For this review, take the finished solid that the model builds, in its own axes (mm). Give positions to 0.01 mm unless a question says otherwise; leave off trailing zeros. Write each loop counter-clockwise with the first axis right and the second up, starting at its lowest first coordinate (ties: lowest second). Pieces come first, ordered by that corner, then holes. Notation, with made-up numbers: (-33.5, 32.5) -> (14.5, 32.5) arc R29 ccw to (14.5, 65.5) -> close; hole circle Ø1 at (43, -15.5). An arc over 180 degrees is marked (long way). Answer as CSV lines item,"result".
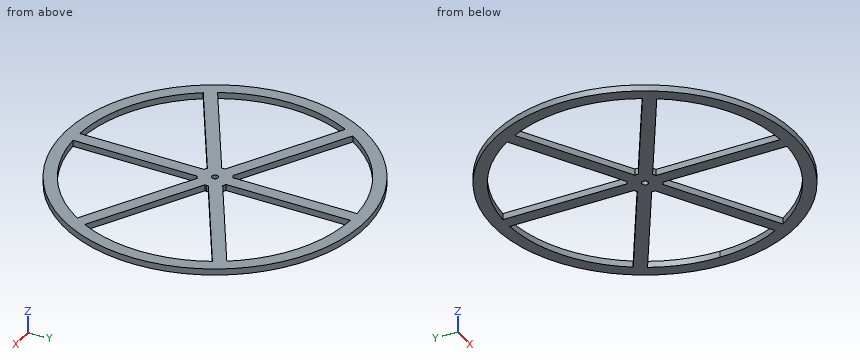
```python
from build123d import *

# Parameters (mm, degrees)
F0_R     = 76.2
F0_R_2   = 1.5875
F1_DEPTH = 3.175


with BuildPart() as f1:
    # F0 (on Top) → F1 (new body)
    with BuildSketch(Plane.XY):
        Circle(F0_R)
        with BuildLine():
            ThreePointArc((62.016851, 32.139271), (67.863464, 16.540035), (69.85, 0))
            ThreePointArc((69.85, 0), (67.863464, -16.540035), (62.016851, -32.139271))
            ThreePointArc((62.016851, -32.139271), (60.491874, -34.925), (58.841851, -37.638532))
            ThreePointArc((58.841851, -37.638532), (34.925, -60.491874), (3.175, -69.777804))
            ThreePointArc((3.175, -69.777804), (0, -69.85), (-3.175, -69.777804))
            ThreePointArc((-3.175, -69.777804), (-34.925, -60.491874), (-58.841851, -37.638532))
            ThreePointArc((-58.841851, -37.638532), (-60.491874, -34.925), (-62.016851, -32.139271))
            ThreePointArc((-62.016851, -32.139271), (-69.85, 0), (-62.016851, 32.139271))
            ThreePointArc((-62.016851, 32.139271), (-60.491874, 34.925), (-58.841851, 37.638532))
            ThreePointArc((-58.841851, 37.638532), (-34.925, 60.491874), (-3.175, 69.777804))
            ThreePointArc((-3.175, 69.777804), (0, 69.85), (3.175, 69.777804))
            ThreePointArc((3.175, 69.777804), (34.925, 60.491874), (58.841851, 37.638532))
            ThreePointArc((58.841851, 37.638532), (60.491874, 34.925), (62.016851, 32.139271))
        make_face(mode=Mode.SUBTRACT)
        with BuildLine():
            Line((-4.712695, 6.38705), (-58.841851, 37.638532))
            ThreePointArc((-58.841851, 37.638532), (-60.491874, 34.925), (-62.016851, 32.139271))
            Line((-62.016851, 32.139271), (-7.887695, 0.887789))
            ThreePointArc((-7.887695, 0.887789), (-6.874077, 3.96875), (-4.712695, 6.38705))
        make_face()
        with BuildLine():
            ThreePointArc((-62.016851, -32.139271), (-60.491874, -34.925), (-58.841851, -37.638532))
            Line((-58.841851, -37.638532), (-4.712695, -6.38705))
            ThreePointArc((-4.712695, -6.38705), (-6.874077, -3.96875), (-7.887695, -0.887789))
            Line((-7.887695, -0.887789), (-62.016851, -32.139271))
        make_face()
        with BuildLine():
            ThreePointArc((7.9375, 0), (7.925039, 0.444592), (7.887695, 0.887789))
            ThreePointArc((7.887695, 0.887789), (6.874077, 3.96875), (4.712695, 6.38705))
            ThreePointArc((4.712695, 6.38705), (3.96875, 6.874077), (3.175, 7.274839))
            Line((3.175, 7.274839), (-3.175, 7.274839))
            ThreePointArc((-3.175, 7.274839), (-3.96875, 6.874077), (-4.712695, 6.38705))
            ThreePointArc((-4.712695, 6.38705), (-6.874077, 3.96875), (-7.887695, 0.887789))
            ThreePointArc((-7.887695, 0.887789), (-7.9375, 0), (-7.887695, -0.887789))
            ThreePointArc((-7.887695, -0.887789), (-6.874077, -3.96875), (-4.712695, -6.38705))
            ThreePointArc((-4.712695, -6.38705), (-3.96875, -6.874077), (-3.175, -7.274839))
            ThreePointArc((-3.175, -7.274839), (0, -7.9375), (3.175, -7.274839))
            ThreePointArc((3.175, -7.274839), (3.96875, -6.874077), (4.712695, -6.38705))
            ThreePointArc((4.712695, -6.38705), (6.874077, -3.96875), (7.887695, -0.887789))
            ThreePointArc((7.887695, -0.887789), (7.925039, -0.444592), (7.9375, 0))
        make_face()
        Circle(F0_R_2, mode=Mode.SUBTRACT)
        with BuildLine():
            ThreePointArc((-3.175, -69.777804), (0, -69.85), (3.175, -69.777804))
            Line((3.175, -69.777804), (3.175, -7.274839))
            ThreePointArc((3.175, -7.274839), (0, -7.9375), (-3.175, -7.274839))
            Line((-3.175, -7.274839), (-3.175, -69.777804))
        make_face()
        with BuildLine():
            ThreePointArc((58.841851, -37.638532), (60.491874, -34.925), (62.016851, -32.139271))
            Line((62.016851, -32.139271), (7.887695, -0.887789))
            ThreePointArc((7.887695, -0.887789), (6.874077, -3.96875), (4.712695, -6.38705))
            Line((4.712695, -6.38705), (58.841851, -37.638532))
        make_face()
        with BuildLine():
            Line((7.887695, 0.887789), (62.016851, 32.139271))
            ThreePointArc((62.016851, 32.139271), (60.491874, 34.925), (58.841851, 37.638532))
            Line((58.841851, 37.638532), (4.712695, 6.38705))
            ThreePointArc((4.712695, 6.38705), (6.874077, 3.96875), (7.887695, 0.887789))
        make_face()
        with BuildLine():
            Line((3.175, 7.274839), (3.175, 69.777804))
            ThreePointArc((3.175, 69.777804), (0, 69.85), (-3.175, 69.777804))
            Line((-3.175, 69.777804), (-3.175, 7.274839))
            ThreePointArc((-3.175, 7.274839), (0, 7.9375), (3.175, 7.274839))
        make_face()
        with BuildLine():
            Line((-3.175, 7.274839), (3.175, 7.274839))
            ThreePointArc((3.175, 7.274839), (0, 7.9375), (-3.175, 7.274839))
        make_face()
    extrude(amount=F1_DEPTH)


solid = f1.part
```
Q1. Add section C-C (z = 2.5). State how many separate pieces and enclosed holes the cut face has, plus the area to 3 significant figures.
Answer block:
separate pieces,"1"
enclosed holes,"7"
area,"5,470 mm2"
Q2. Add section D-D (y = -52.5). Write out the cut boundary in (x, z) (3 decimals), plus the area to 3 significant figures.
Answer block:
outline,"(-55.229, 0) -> (-46.074, 0) -> (-46.074, 3.175) -> (-55.229, 3.175) -> close; (-3.175, 0) -> (3.175, 0) -> (3.175, 3.175) -> (-3.175, 3.175) -> close; (46.074, 0) -> (55.229, 0) -> (55.229, 3.175) -> (46.074, 3.175) -> close"
area,"78.3 mm2"
Q3. Clearance check with flat-ended pins moving along their axes: pin 1 (1.5 mm diameter, centred on y = 48.5, z = 2.5, fed in from +X); pin 2 (1.6 mm diameter, centred on y = -41.5, z = 1.5, fed in from -X); pin 3 (1.6 mm diameter, centred on y = 23.5, z = 2, fed in from -X); pin 4 (2.5 mm diameter, centred on x = 0, y = 0, fed in from +Z). State where each tip first meets the part, or that it passes through.
Answer block:
pin 1,"stops at x = 59.38"
pin 2,"stops at x = -64.42"
pin 3,"stops at x = -72.74"
pin 4,"passes through"
Q4. Add section B-B (x = 40.5). Write out the cut boundary in (y, z) (3 decimals).
Answer block:
outline,"(-64.546, 0) -> (-56.91, 0) -> (-56.91, 3.175) -> (-64.546, 3.175) -> close; (-27.049, 0) -> (-19.717, 0) -> (-19.717, 3.175) -> (-27.049, 3.175) -> close; (19.717, 0) -> (27.049, 0) -> (27.049, 3.175) -> (19.717, 3.175) -> close; (56.91, 0) -> (64.546, 0) -> (64.546, 3.175) -> (56.91, 3.175) -> close"
Q5. Add section A-A (y = 13). Write out the cut boundary in (x, z) (3 decimals), plus the area to 3 significant figures.
Answer block:
outline,"(-75.083, 0) -> (-68.63, 0) -> (-68.63, 3.175) -> (-75.083, 3.175) -> close; (-28.867, 0) -> (-16.167, 0) -> (-16.167, 3.175) -> (-28.867, 3.175) -> close; (-3.175, 0) -> (3.175, 0) -> (3.175, 3.175) -> (-3.175, 3.175) -> close; (16.167, 0) -> (28.867, 0) -> (28.867, 3.175) -> (16.167, 3.175) -> close; (68.63, 0) -> (75.083, 0) -> (75.083, 3.175) -> (68.63, 3.175) -> close"
area,"142 mm2"
Q6. To check wall thickness, follow probe 1 along X at (y, z) = (-36, 1.55) (3 decimals); probe 2 along X at (y, z) = (13.5, 1.8) (3 decimals); probe 3 along X at (y, z) = (60.5, 2) (3 decimals). State the ranges of each line that lie inside material, in increasing order. Write a range as [from, to].
Answer block:
probe 1,"x = [-67.16, -56.004], [-3.175, 3.175], [56.004, 67.16]"
probe 2,"x = [-74.995, -68.533], [-29.733, -17.033], [-3.175, 3.175], [17.033, 29.733], [68.533, 74.995]"
probe 3,"x = [-46.327, -34.911], [-3.175, 3.175], [34.911, 46.327]"
